Source: CAD feature listing. Evaluate the final solid. Frame: model axes, mm. A direction names the side the tool comes from. Give positions to 0.01 mm unless a question says otherwise; leave off trailing zeros. Loops run counter-clockwise (first coordinate to the right, second up) from the corner with the lowest first, then second, coordinate; pieces in that order, holes last. Notation, with made-up numbers: M 67,83 L 100,83 A22 ccw 100,114 Z; hole C 74.5,-23 d6. An arc over 180 degrees is marked long. Put each result on its own line as item: value.
from build123d import *

# Parameters (mm, degrees)
BOSS_EXTRUDE1_DEPTH = 4
SKETCH2_R           = 11
BOSS_EXTRUDE2_DEPTH = 25.4
SKETCH3_R           = 8
CUT_EXTRUDE1_DEPTH  = 22.86
CUT_EXTRUDE2_DEPTH  = 22.86
SKETCH5_R           = 3
SKETCH5_W           = 22.8
SKETCH5_H           = 12.6
CUT_EXTRUDE3_DEPTH  = 4
BOSS_EXTRUDE3_DEPTH = 10
SKETCH7_W           = 4.84
SKETCH7_H           = 6.056432248
CUT_EXTRUDE4_DEPTH  = 10


with BuildPart() as part:
    # Sketch1 → Boss-Extrude1 (new body)
    with BuildSketch(Plane(origin=(0, 0, 0), x_dir=(1, 0, 0), z_dir=(0, 1, 0))):
        Polygon((76.2, 0), (-38.1, 65.991135768), (-38.1, -65.991135768), align=None)
    extrude(amount=BOSS_EXTRUDE1_DEPTH)

    # Sketch2 → Boss-Extrude2 (add)
    with BuildSketch(Plane(origin=(0, 4, 0), x_dir=(1, 0, 0), z_dir=(0, 1, 0))):
        with Locations((20.32, 0)):
            Circle(SKETCH2_R)
        with Locations((-10.16, 17.597636205)):
            Circle(SKETCH2_R)
        with Locations((-10.16, -17.597636205)):
            Circle(SKETCH2_R)
    extrude(amount=BOSS_EXTRUDE2_DEPTH)

    # Sketch3 → Cut-Extrude1 (cut)
    with BuildSketch(Plane(origin=(0, 29.4, 0), x_dir=(1, 0, 0), z_dir=(0, 1, 0))):
        with Locations((-10.16, 17.597636205)):
            Circle(SKETCH3_R)
        with Locations((20.32, 0)):
            Circle(SKETCH3_R)
        with Locations((-10.16, -17.597636205)):
            Circle(SKETCH3_R)
    extrude(amount=-CUT_EXTRUDE1_DEPTH, mode=Mode.SUBTRACT)

    # Sketch4 → Cut-Extrude2 (cut)
    with BuildSketch(Plane(origin=(0, 4, 0), x_dir=(1, 0, 0), z_dir=(0, 1, 0))):
        Polygon((-38.1, 65.991135768), (-1.726933041, 44.991135768), (-38.1, 23.991135768), align=None)
        Polygon((-38.1, -65.991135768), (-1.726933041, -44.991135768), (-38.1, -23.991135768), align=None)
        Polygon((76.2, 0), (39.826933041, -21), (39.826933041, 21), align=None)
    extrude(amount=-CUT_EXTRUDE2_DEPTH, mode=Mode.SUBTRACT)

    # Sketch5 → Cut-Extrude3 (cut)
    with BuildSketch(Plane(origin=(0, 0, 0), x_dir=(-1, 0, 0), z_dir=(0, -1, 0))):
        with Locations((-7.753054986, -14.0369452)):
            Circle(SKETCH5_R)
        with Locations((4.5, 0)):
            Rectangle(SKETCH5_W, SKETCH5_H)
    extrude(amount=-CUT_EXTRUDE3_DEPTH, mode=Mode.SUBTRACT)

    # Sketch6 → Boss-Extrude3 (add)
    with BuildSketch(Plane(origin=(0, 4, 0), x_dir=(1, 0, 0), z_dir=(0, 1, 0))):
        Polygon((-6.061319385, 26.273055398), (-10.196194275, 33.309488143), (-14.22248634, 26.210365074), align=None)
        Polygon((-15.553445676, 10.019414489), (-19.902730969, 18.097665314), (-24.724058755, 10.291948349), align=None)
        Polygon((4.666083615, 11.839822271), (-0.028890737, 18.987902238), (-3.871822401, 11.347895195), align=None)
        Polygon((25.015642032, 8.329035834), (20.285301804, 16.40202737), (15.659056164, 8.268936796), align=None)
        Polygon((33.276250833, -7.973152462), (30.121872493, -1.379377193), (25.988684773, -7.408036604), align=None)
        Polygon((15.659056164, -7.973152462), (10.527139401, -1.011359201), (7.064007962, -8.936626119), align=None)
        Polygon((-15.553445676, -9.963714295), (-23.645110056, -9.611162466), (-19.904596706, -16.795025293), align=None)
        Polygon((-5.170207238, -25.158366131), (-14.52400497, -26.588552978), (-8.608527963, -33.974086013), align=None)
        Polygon((-0.901197828, -18.18923766), (4.614077612, -11.758341231), (-3.712879784, -10.197420805), align=None)
    extrude(amount=BOSS_EXTRUDE3_DEPTH)

    # Sketch7 → Cut-Extrude4 (cut)
    with BuildSketch(Plane(origin=(0, 4, 0), x_dir=(1, 0, 0), z_dir=(0, 1, 0))):
        with Locations((6.9, 0)):
            Rectangle(SKETCH7_W, SKETCH7_H)
    extrude(amount=-CUT_EXTRUDE4_DEPTH, mode=Mode.SUBTRACT)


solid = part.part
1. Section query A-A (y = 10.25). State how many separate pieces and enclosed holes the cut face has, plus the area to 3 significant figures.
Found:
separate pieces: 3
enclosed holes: 3
area: 673 mm^2
2. Section query D-D (z = -15). Output: boundary loops of the cut face in (x, y).
Found:
outline: M -38.1,0 L 39.83,0 L 39.83,4 L 21.11,4 L 21.11,14 L 19.49,14 L 19.49,4 L 2.59,4 L 2.59,14 L 0.53,14 L 0.53,29.4 L -2.59,29.4 L -2.59,6.54 L -17.73,6.54 L -17.73,29.4 L -20.85,29.4 L -20.85,14 L -21.82,14 L -21.82,4 L -38.1,4 Z
3. Section query C-C (x = 19). Output: boundary loops of the cut face in (y, z), plus the area to 3 significant figures.
Found:
outline: M 0,-33.02 L 4,-33.02 L 4,-14.14 L 14,-14.14 L 14,-10.92 L 29.4,-10.92 L 29.4,-7.89 L 6.54,-7.89 L 6.54,7.89 L 29.4,7.89 L 29.4,10.92 L 4,10.92 L 4,33.02 L 0,33.02 Z
area: 490 mm^2
4. Draft query along Z for faces 6 (the flat face through (9, 14, 7)), 7 (the flat face through (-8.67, 8.93, -30.71)), 8 (the cylindrical face through (-2.53, 18.13, 15.19)). Return one class per face: pulls with the +Z half, pulls with the -Z half, needs draft (parallel to the pull), parting line crosses it, or undercut.
Found:
face 6: needs draft
face 7: pulls with the -Z half
face 8: undercut
5. Section query B-B (y = 5.5). Output: boundary loops of the cut face in (x, z).
Found:
outline: M -24.72,-10.29 L -21.07,-16.21 A11 ccw -13.09,-28.2 L -10.2,-33.31 L -7.19,-28.19 A11 ccw 0.84,-17.67 L 4.67,-11.84 L -1,-11.51 A11 ccw -18.21,-10.1 Z; M -23.65,9.61 L -17.98,9.86 A11 ccw -1.69,10.58 L 4.61,11.76 L 0.76,16.25 A11 ccw -6.23,27.87 L -8.61,33.97 L -13.28,28.15 A11 ccw -20.85,14.99 Z; M 7.06,8.94 L 9.71,2.89 A11 ccw 16.9,-10.46 L 20.29,-16.4 L 23.78,-10.44 A11 ccw 30.9,3.01 L 33.28,7.97 L 28.29,7.59 A11 ccw 13.06,8.26 Z
6. Material intervals for line 1 (Z direction, x = -10, y = 25); line 2 (Z direction, x = -8.5, y = 16.5); line 3 (X direction, y = 12.5, z = 0), sorted ascending. Write a range as from..to.
Found:
line 1: -28.6..-25.6, -9.6..-6.6, 6.6..9.6, 25.6..28.6
line 2: -28.47..-25.42, -9.77..-6.72, 6.72..9.77, 25.42..28.47
line 3: 9.32..12.32, 28.32..31.32
7. Access query for faces 1 (the flat face through (-20.771, 8.93, 9.736)), 2 (the flat face through (-4, 2, -6.3)), 3 (the flat face through (-7.435, 8.93, 30.965)), 4 (the flat face through (-11.625, 8.93, -30.79)), 5 (the flat face through (18.618, 8.93, -13.471)). Directions: +Z, -Z, +X, -X, +Y, -Y. A direction counts if a zero-diameter tool reaches every point of the face in a straight line with its end or side. Return the directions, or none.
Found:
face 1: +Y
face 2: +Y, -Y
face 3: +Z, +X, +Y
face 4: -Z, -X, +Y
face 5: -Z, +Y
8. Contact query for flat-ended pins moving along their axis: P1, Ø4, axis at x = -9.5, z = -32, coming from the +Y side; P2, Ø5, axis at x = 17.5, z = -2.5, coming from the +Y side; P3, Ø1.2, axis at x = -6, y = 1, coming from the -Z side. Output: stop coordinate, or through.
Found:
P1: y = 14
P2: y = 6.54
P3: z = -42.87
